from build123d import *

# Parameters (mm, degrees)
ESQUISSE1_W                  = 28
ESQUISSE1_H                  = 25
BOSS_EXTRU_1_DEPTH           = 4
ESQUISSE2_W                  = 28
ESQUISSE2_H                  = 10
BOSS_EXTRU_2_DEPTH           = 10
ENL_V_MAT_EXTRU_1_DEPTH      = 41.062451248
ENL_V_MAT_EXTRU_1_DEPTH_BACK = 41.062451248
ESQUISSE3_R                  = 1.75
CONG_1_R                     = 3
ESQUISSE4_W                  = 12
ESQUISSE4_H                  = 16
ENL_V_MAT_EXTRU_2_DEPTH      = 10
ENL_V_MAT_EXTRU_3_DEPTH      = 39.845849199
ENL_V_MAT_EXTRU_3_DEPTH_BACK = 39.845849199
ESQUISSE5_R                  = 2
CHANFREIN1_SIZE              = 2
CONG_2_R                     = 10


with BuildPart() as part:
    # Esquisse1 → Boss.-Extru.1 (new body)
    with BuildSketch(Plane.XY):
        with Locations((14, 12.5)):
            Rectangle(ESQUISSE1_W, ESQUISSE1_H)
    extrude(amount=BOSS_EXTRU_1_DEPTH)

    # Esquisse2 → Boss.-Extru.2 (add)
    with BuildSketch(Plane.XY.offset(4)):
        with Locations((14, 12.5)):
            Rectangle(ESQUISSE2_W, ESQUISSE2_H)
    extrude(amount=BOSS_EXTRU_2_DEPTH)

    # Esquisse3 → Enlèv. mat.-Extru.1 (cut, two sides: drawn at the far end of the back side and taken through both)
    with BuildSketch(Plane(origin=(28, 0, 0), x_dir=(0, 0, -1), z_dir=(1, 0, 0)).offset(-ENL_V_MAT_EXTRU_1_DEPTH_BACK)):
        with Locations((-9, 12.5)):
            Circle(ESQUISSE3_R)
    extrude(amount=ENL_V_MAT_EXTRU_1_DEPTH + ENL_V_MAT_EXTRU_1_DEPTH_BACK, mode=Mode.SUBTRACT)

    # Congé1
    cong_1_edges = [part.edges().sort_by_distance(p)[0] for p in [
        (14, 17.5, 4),
        (14, 7.5, 4),
        (14, 17.5, 14),
        (14, 7.5, 14),
    ]]
    fillet(cong_1_edges, radius=CONG_1_R)

    # Esquisse4 → Enlèv. mat.-Extru.2 (cut)
    with BuildSketch(Plane.XY.offset(4)):
        with Locations((14, 12.5)):
            Rectangle(ESQUISSE4_W, ESQUISSE4_H)
    extrude(amount=ENL_V_MAT_EXTRU_2_DEPTH, mode=Mode.SUBTRACT)

    # Esquisse5 → Enlèv. mat.-Extru.3 (cut, two sides: drawn at the far end of the back side and taken through both)
    with BuildSketch(Plane.XY.offset(4).offset(-ENL_V_MAT_EXTRU_3_DEPTH_BACK)):
        with Locations((14, 20.5)):
            Circle(ESQUISSE5_R)
        with Locations(Location((14, 4.5, 0), (0, 0, 180))):
            Circle(ESQUISSE5_R)
    extrude(amount=ENL_V_MAT_EXTRU_3_DEPTH + ENL_V_MAT_EXTRU_3_DEPTH_BACK, mode=Mode.SUBTRACT)

    # Chanfrein1
    chanfrein1_edges = [part.edges().sort_by_distance(p)[0] for p in [
        (16, 4.5, 4),
        (12, 20.5, 4),
    ]]
    chamfer(chanfrein1_edges, length=CHANFREIN1_SIZE)

    # Congé2
    cong_2_edges = [part.edges().sort_by_distance(p)[0] for p in [
        (28, 0, 2),
        (0, 0, 2),
        (0, 25, 2),
        (28, 25, 2),
    ]]
    fillet(cong_2_edges, radius=CONG_2_R)


solid = part.part
Design review of the part built by this model. Coordinates are the model's own, in mm. A direction names the side the tool comes from. Give positions to 0.01 mm unless a question says otherwise; leave off trailing zeros. Order: outer loops, then holes, each group sorted by start corner. A loop starts at its lowest first (then second) coordinate and runs counter-clockwise, first axis right, second up. Notation, with made-up numbers: (50, 46.5) - (75, 46.5) arc R18 cw to (75, 73.5) - close; hole circle Ø10 at (-10.75, 1). An arc over 180 degrees is marked (long way). Write item = value, one per line. Start each with the question number.
Q1. Mouldability with a two-part tool opening along Y and no side actions: class faces 6 (the face through (24, 7.5, 9)), 7 (the face through (4.21, 18.4, 4.86)), 8 (the face through (28, 12, 7)), 9 (the face through (23.944, 13.026, 7.331)) as released by +Y, released by -Y, zero draft, split by the parting line, or undercut.
Q2. Clearance check with flat-ended pins moving along their axes: pin 1 Ø8 at (x, z) = (6, 6) entering from +Y; pin 2 Ø4.5 at (x, z) = (24, 10) entering from +Y; pin 3 Ø4.5 at (x, z) = (25.5, 9) entering from -Y. State where each tip first meets the part, or that it passes through.
Q3. We need section B-B on z = 2.5. State the section outline as (x, y) points.
Q4. Tool access review of faces 1 (the face through (14, 13, 4)), 2 (the face through (15.6, 5.7, 1)), 3 (the face through (24, 17.5, 9)), 4 (the face through (20, 10.6, 8.9)), 5 (the face through (23.9, 6.6, 4.86)): name each direction out of +Z, -Z, +X, -X, +Y, -Y from which nothing blocks a thin tool from reaching the whole face with its end or side.
Q5. We need section A-A on x = 14. State the section outline as (y, z) points.
Q6. To check wall thickness, follow L1, parallel to Y at x = 14, z = 1.05; L2, parallel to Y at x = 5.75, z = 9; L3, parallel to X at y = 20.5, z = 1.1. State the ranges of each line that lie inside material, in increasing order. Write a range as from..to.
Q7. We need section C-C on z = 9. State the section outline as (x, y) points.
Q8. We need section D-D on x = 6.25. State the section outline as (y, z) points.
Working result:
q1.face_6 = released by -Y
q1.face_7 = released by +Y
q1.face_8 = zero draft
q1.face_9 = undercut
q2.pin_1 = 24.99
q2.pin_2 = 17.5
q2.pin_3 = 7.49
q3.outline = (0, 10) arc R10 ccw to (10, 0) - (18, 0) arc R10 ccw to (28, 10) - (28, 15) arc R10 ccw to (18, 25) - (10, 25) arc R10 ccw to (0, 15) - close; hole circle Ø5 at (14, 4.5); hole circle Ø5 at (14, 20.5)
q4.face_1 = +Z
q4.face_2 = +Z, -Z
q4.face_3 = +Z, +X, -X, +Y
q4.face_4 = +Z, +Y, -Y
q4.face_5 = +Z, +X, -X, -Y
q5.outline = (0, 0) - (2.5, 0) - (2.5, 2) - (0.5, 4) - (0, 4) - close; (6.5, 0) - (18.5, 0) - (18.5, 2) - (16.5, 4) - (8.5, 4) - (6.5, 2) - close; (22.5, 0) - (25, 0) - (25, 4) - (24.5, 4) - (22.5, 2) - close
q6.L1 = 0..2.5, 6.5..18.5, 22.5..25
q6.L2 = 7.5..10.75, 14.25..17.5
q6.L3 = 1.65..12, 16..26.35
q7.outline = (0, 10) arc R10 ccw to (0.32, 7.5) - (8, 7.5) - (8, 10.75) - (0, 10.75) - close; (0, 14.25) - (8, 14.25) - (8, 17.5) - (0.32, 17.5) arc R10 ccw to (0, 15) - close; (20, 7.5) - (27.68, 7.5) arc R10 ccw to (28, 10) - (28, 10.75) - (20, 10.75) - close; (20, 14.25) - (28, 14.25) - (28, 15) arc R10 ccw to (27.68, 17.5) - (20, 17.5) - close
q8.outline = (0.73, 0) - (24.27, 0) - (24.27, 4) - (20.5, 4) arc R3 cw to (17.5, 7) - (17.5, 11) arc R3 ccw to (14.5, 14) - (10.5, 14) arc R3 ccw to (7.5, 11) - (7.5, 7) arc R3 cw to (4.5, 4) - (0.73, 4) - close; hole circle Ø3.5 at (12.5, 9)
